```python
from build123d import *

# Parameters (mm, degrees)
F0_R     = 1
F0_R_2   = 2
F1_DEPTH = 1
F2_R     = 2


with BuildPart() as f1:
    # F0 (on Top) → F1 (new body)
    with BuildSketch(Plane.XY):
        with BuildLine():
            ThreePointArc((-2.5, 28.1224989992), (-4, 25), (-2.5, 21.8775010008))
            Line((-2.5, 21.8775010008), (-2.5, 28.1224989992))
        make_face()
        with BuildLine():
            ThreePointArc((1.9364916731, 28.5), (0, 29), (-1.9364916731, 28.5))
            Line((-1.9364916731, 28.5), (1.9364916731, 28.5))
        make_face()
        with BuildLine():
            Line((3.2255519271, 27.3655474558), (3.8851082618, 24.0481944557))
            ThreePointArc((3.8851082618, 24.0481944557), (3.9711731923, 24.5206426422), (4, 25))
            ThreePointArc((4, 25), (3.8014607527, 26.2445465624), (3.2255519271, 27.3655474558))
        make_face()
        with BuildLine():
            ThreePointArc((0, -8.5), (-1.2640556872, -8.4054841157), (-2.5, -8.1240384046))
            Line((-2.5, -8.1240384046), (-2.5, -8.5))
            Line((-2.5, -8.5), (0, -8.5))
        make_face()
        with BuildLine():
            ThreePointArc((0, 4), (4, 0), (0, -4))
            Line((0, -4), (-2.5, -4))
            Line((-2.5, -4), (-2.5, -8.1240384046))
            ThreePointArc((-2.5, -8.1240384046), (-1.2640556872, -8.4054841157), (0, -8.5))
            ThreePointArc((0, -8.5), (6.5703494482, -5.3926346185), (8.3368220918, 1.6575274991))
            Line((8.3368220918, 1.6575274991), (3.8851082618, 24.0481944557))
            ThreePointArc((3.8851082618, 24.0481944557), (1.2874815505, 21.2128650332), (-2.5, 21.8775010008))
            Line((-2.5, 21.8775010008), (-2.5, 4))
            Line((-2.5, 4), (0, 4))
        make_face()
        with Locations((0, -6)):
            Circle(F0_R, mode=Mode.SUBTRACT)
        with Locations((0, 6)):
            Circle(F0_R, mode=Mode.SUBTRACT)
        with Locations((4.2426406871, -4.2426406871)):
            Circle(F0_R, mode=Mode.SUBTRACT)
        with Locations((6, 0)):
            Circle(F0_R, mode=Mode.SUBTRACT)
        with Locations((4.2426406871, 4.2426406871)):
            Circle(F0_R, mode=Mode.SUBTRACT)
        with BuildLine():
            Line((-2.5, 28.1224989992), (-2.5, 21.8775010008))
            ThreePointArc((-2.5, 21.8775010008), (1.2874815505, 21.2128650332), (3.8851082618, 24.0481944557))
            Line((3.8851082618, 24.0481944557), (3.2255519271, 27.3655474558))
            ThreePointArc((3.2255519271, 27.3655474558), (2.6426159721, 28.002762199), (1.9364916731, 28.5))
            Line((1.9364916731, 28.5), (-1.9364916731, 28.5))
            ThreePointArc((-1.9364916731, 28.5), (-2.2262617418, 28.3232151085), (-2.5, 28.1224989992))
        make_face()
        with Locations((0, 25)):
            Circle(F0_R_2, mode=Mode.SUBTRACT)
    extrude(amount=F1_DEPTH)

    # F2
    f2_edges = [f1.edges().sort_by_distance(p)[0] for p in [
        (-2.5, 4, 0.5),
        (-2.5, -4, 0.5),
        (-2.5, -8.5, 0.5),
        (-2.5, 21.877501, 0.5),
        (3.885108, 24.048194, 0.5),
    ]]
    fillet(f2_edges, radius=F2_R)


solid = f1.part
```
Check sheet for the modelled part. Datum: model origin and axes. Units: mm. A direction names the side the tool comes from. Round coordinates to 2 decimals unless told otherwise and drop trailing zeros. Loops run counter-clockwise (first coordinate to the right, second up) from the corner with the lowest first, then second, coordinate; pieces in that order, holes last. Notation, with made-up numbers: (-30, 79.25) - (6, 79.25) arc R18 ccw to (6, 105.25) - close; hole circle Ø1 at (78.5, 80). An arc over 180 degrees is marked (long way). Write item = value, one per line. Start each with the question number.
Q1. Access from +Z, -Z, +X, -X, +Y, -Y to the whole of each face (thin tool, end or side, straight path). Record for faces 1 (the face through (-2.5, 13.6, 0.5)), 2 (the face through (-1.9, -4.57, 0.51)), 3 (the face through (3.45, 3.63, 0.49)).
Q2. Section check D-D (y = 9.5). Record the boundary of the cut face in (x, z), plus the area to 3 significant figures.
Q3. Section check B-B (x = 6). Record the boundary of the cut face in (y, z), plus the area to 3 significant figures.
Q4. Section check A-A (y = 0). Record the boundary of the cut face in (x, z).
Q5. Thickness scan on L1, parallel to Y at x = 1.5, z = 0.1; L2, parallel to Y at x = 2.25, z = 0.9; L3, parallel to Y at x = 3, z = 0.4. Record the ranges inside material, lowest first.
Q6. Release check for a two-part mould opening along X. For faces 4 (the face through (-1.93, -7.9, 0.51)), 5 (the face through (2, 11, 1)), 6 (the face through (3.506, -3.567, 0.493)), 7 (the face through (-0.13, -5.01, 0.49)) record: pulls with the +X half, pulls with the -X half, needs draft (parallel to the pull), parting line crosses it, or undercut.
Q7. Section check C-C (z = 0.2). Record the boundary of the cut face in (x, y), plus the area to 3 significant figures.
Derived:
q1.face_1 = +Z, -Z, -X, -Y
q1.face_2 = +Z, -Z, -X
q1.face_3 = +Z, -Z
q2.outline = (-2.5, 0) - (6.78, 0) - (6.78, 1) - (-2.5, 1) - close
q2.area = 9.28 mm^2
q3.outline = (-6.02, 0) - (-1, 0) - (-1, 1) - (-6.02, 1) - close; (1, 0) - (13.41, 0) - (13.41, 1) - (1, 1) - close
q3.area = 17.4 mm^2
q4.outline = (4, 0) - (5, 0) - (5, 1) - (4, 1) - close; (7, 0) - (8.5, 0) - (8.5, 1) - (7, 1) - close
q5.L1 = -8.37 to -3.71, 3.71 to 23.68, 26.32 to 28.71
q5.L2 = -8.2 to -3.31, 3.31 to 28.31
q5.L3 = -7.95 to -2.65, 2.65 to 27.65
q6.face_4 = pulls with the -X half
q6.face_5 = needs draft
q6.face_6 = undercut
q6.face_7 = undercut
q7.outline = (-3, 22.35) arc R2 cw to (-2.5, 21.03) - (-2.5, 6) arc R2 ccw to (-0.5, 4) - (0, 4) arc R4 cw to (0, -4) - (-0.5, -4) arc R2 ccw to (-2.5, -6) - (-2.5, -6.5) arc R2 ccw to (-0.5, -8.5) - (0, -8.5) arc R8.5 ccw to (8.34, 1.66) - (3.96, 23.66) arc R2 cw to (3.95, 24.37) arc R4 ccw (long way) to start; hole circle Ø4 at (0, 25); hole circle Ø2 at (0, -6); hole circle Ø2 at (0, 6); hole circle Ø2 at (4.24, -4.24); hole circle Ø2 at (4.24, 4.24); hole circle Ø2 at (6, 0)
q7.area = 248 mm^2
